Study the drawing (mm; zero at the part's minimum x, y, z) and answer. A direction names the side the tool comes from. Round coordinates to 2 decimals unless told otherwise and drop trailing zeros. Order: outer loops, then holes, each group sorted by start corner. A loop starts at its lowest first (then second) coordinate and runs counter-clockwise, first axis right, second up. Notation, with made-up numbers: (-9.5, 43) - (0.5, 43) arc R34 ccw to (0.5, 75) - close; hole circle Ø6 at (66, 89.5). An arc over 180 degrees is marked (long way). Put each result on its own line as item: value.
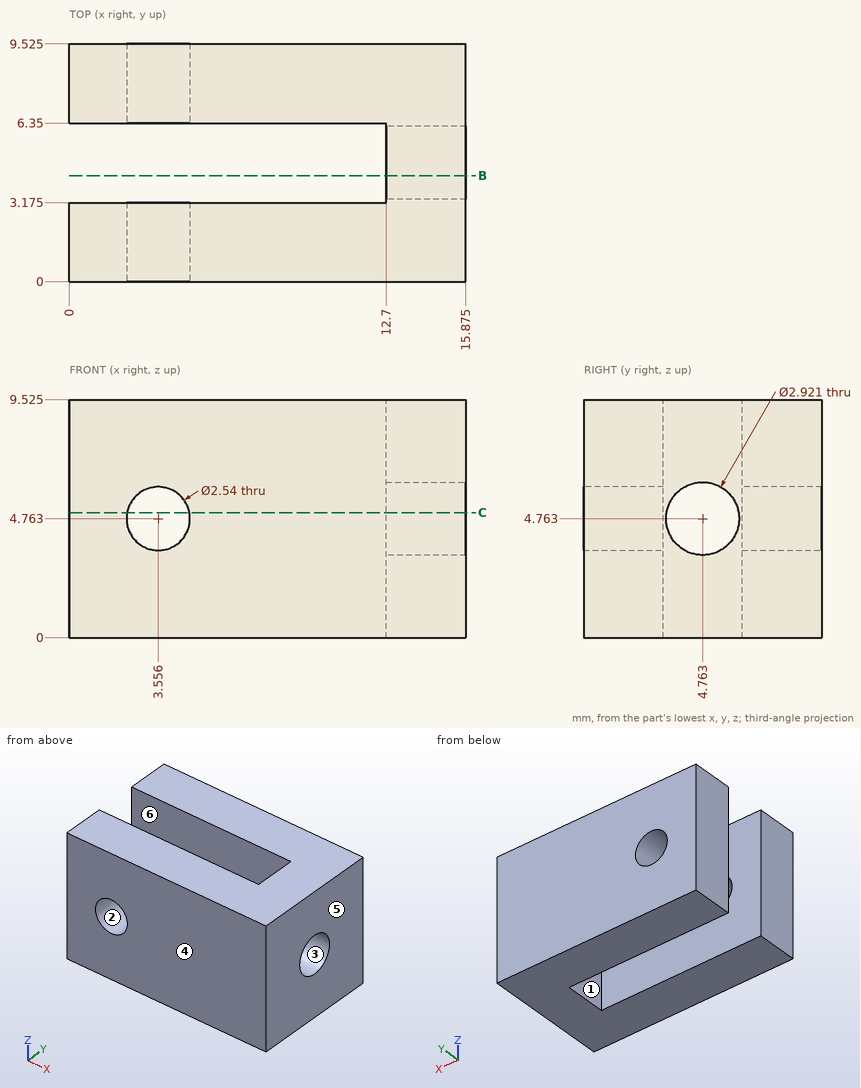
1) Straight lines are drawn through the part: L1, parallel to X at y = 5, z = 3.25 (1 decimal); L2, parallel to Y at x = 15.25, z = 4.75 (1 decimal); L3, parallel to Z at x = 4.5, y = 8.5 (1 decimal). For each, find the intervals that lie inside material, in ascending order. Write a range as from..to.
Findings below:
L1: x = 12.7..15.9
L2: y = 0..3.3, 6.2..9.5
L3: z = 0..3.9, 5.6..9.5
2) A cutting plane is placed at C-C on z = 5. Give the number of separate pieces and of enclosed holes in the cut face.
Findings below:
separate pieces: 4
enclosed holes: 0
3) Given pin 1 Ø5 at (x, y) = (8, 3) entering from -Z; pin 2 Ø2.5 at (y, z) = (4.5, 4.5) entering from -X, each flat-ended and moving along its own axis, determine where each tip first touches the part or whether it passes through.
Findings below:
pin 1: stops at z = 0
pin 2: stops at x = 12.7
4) For the marked faces 1 and 2, determine the directions among +Z, -Z, +X, -X, +Y, -Y from which every point of the face is accessible in a straight line to the end or side of a thin tool.
Findings below:
face 1: +Z, -Z, -X
face 2: +Y, -Y
5) A cutting plane is placed at B-B on y = 4.25. Write down the section's boundary in (x, z) (1 decimal).
Findings below:
outline: (12.7, 0) - (15.9, 0) - (15.9, 3.4) - (12.7, 3.4) - close; (12.7, 6.1) - (15.9, 6.1) - (15.9, 9.5) - (12.7, 9.5) - close
6) For a pull along Y with two mould halves and no side action, classify the marked faces 3, 4, 5 and 6 as pulls with the +Y half, pulls with the -Y half, needs draft (parallel to the pull), parting line crosses it, or undercut.
Findings below:
face 3: undercut
face 4: pulls with the -Y half
face 5: needs draft
face 6: undercut
